Verification items for the finished model (mm, model axes). Face numbers are marked on the shaded views. A direction names the side the tool comes from. Give positions to 0.01 mm unless a question says otherwise; leave off trailing zeros. Loops run counter-clockwise (first coordinate to the right, second up) from the corner with the lowest first, then second, coordinate; pieces in that order, holes last. Notation, with made-up numbers: M 10,12.25 L 25,12.25 A25 cw 25,32.25 Z; hole C -27.75,7 d2. An arc over 180 degrees is marked long. Write each question's results on one line, items separated by ' | '. Start each with the question number.
Autodesk Inventor part; units mm, degrees
ref_plane "YZ Plane" through (0, 0, 0) normal (1, 0, 0) x (0, 1, 0)
ref_plane "XZ Plane" through (0, 0, 0) normal (0, 1, 0) x (-1, 0, 0)
ref_plane "XY Plane" through (0, 0, 0) normal (0, 0, 1) x (1, 0, 0)
sketch "Sketch1" plane through (0, 0, 0) normal (0, 1, 0) x (-1, 0, 0)
  circle A0 centre (0, 0) radius 30.48
  dimension "d0" = 60.96
extrude "Extrusion1" add sketch "Sketch1" along normal blind 355.6
sketch "Sketch2" plane through (0, 0, 0) normal (0, 1, 0) x (-1, 0, 0)
  circle A0 centre (0, 0) radius 33.98
  circle A1 centre (0, 0) radius 30.48
  dimension "d3" = 3.5
extrude "Extrusion2" add sketch "Sketch2" along normal mid plane 50.8
sketch "Sketch3" plane through (0, 355.6, 0) normal (0, 1, 0) x (1, 0, 0)
  circle A0 centre (0, 0) radius 25.4
  dimension "d6" = 50.8
extrude "Extrusion3" cut sketch "Sketch3" against normal through all
properties part number "Water Sensor Shaft" material "PVC-Piping"
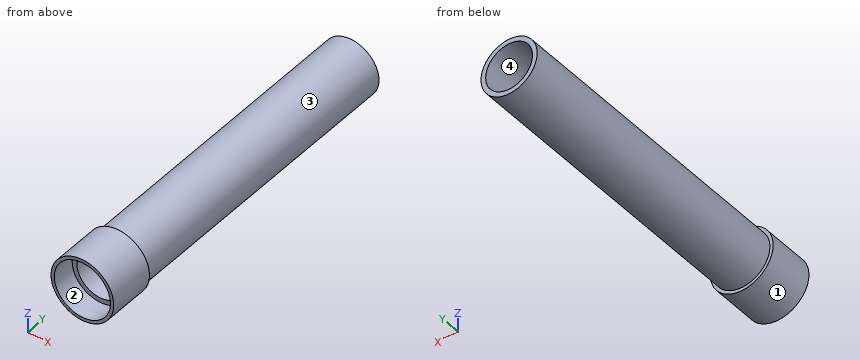
1. Release check for a two-part mould opening along Z. For the marked faces 3 and 4 record: released by +Z, released by -Z, zero draft, split by the parting line, or undercut.
2. Thickness scan on probe 1 along Z at (x, y) = (0, 98); probe 2 along Z at (x, y) = (0, -16); probe 3 along Y at (x, z) = (-23, 14). Record the ranges inside material, lowest first.
3. Set-up check for the marked faces 1 and 2: record each of +Z, -Z, +X, -X, +Y, -Y from which the full face is reachable in a straight line by a thin tool's end or side.
4. Section check B-B, the plane z = -17. Record the boundary of the cut face in (x, y), plus the area to 3 significant figures.
5. Depth check by flat-ended pin: pin 1 Ø6 at (y, z) = (262, 6) entering from +X; pin 2 Ø1.5 at (x, y) = (-9.5, 58) entering from +Z; pin 3 Ø8 at (y, z) = (142, -1.5) entering from +X. Enter the tip coordinate at first touch or a pass-through.
6. Section check C-C, the plane y = 132. Record the boundary of the cut face in (x, z).
7. Section check A-A, the plane x = 0. Record the boundary of the cut face in (y, z).
Filled sheet:
1) face 3: split by the parting line | face 4: undercut
2) probe 1: -30.48 to -25.4, 25.4 to 30.48 | probe 2: -33.98 to -30.48, 30.48 to 33.98 | probe 3: 0 to 355.6
3) face 1: +Y, -Y | face 2: -Y
4) outline: M -29.42,-25.4 L -25.3,-25.4 L -25.3,0 L -18.87,0 L -18.87,355.6 L -25.3,355.6 L -25.3,25.4 L -29.42,25.4 Z; M 18.87,0 L 25.3,0 L 25.3,-25.4 L 29.42,-25.4 L 29.42,25.4 L 25.3,25.4 L 25.3,355.6 L 18.87,355.6 Z | area: 4,990 mm2
5) pin 1: x = 30.33 | pin 2: z = 29.2 | pin 3: x = 30.48
6) outline: C 0,0 d60.96; hole C 0,0 d50.8
7) outline: M -25.4,-33.98 L 25.4,-33.98 L 25.4,-30.48 L 355.6,-30.48 L 355.6,-25.4 L 0,-25.4 L 0,-30.48 L -25.4,-30.48 Z; M -25.4,30.48 L 0,30.48 L 0,25.4 L 355.6,25.4 L 355.6,30.48 L 25.4,30.48 L 25.4,33.98 L -25.4,33.98 Z
